Geometry check sheet. Reference: the model listing, model coordinates, mm. A direction names the side the tool comes from. Give positions to 0.01 mm unless a question says otherwise; leave off trailing zeros. Write each loop counter-clockwise with the first axis right and the second up, starting at its lowest first coordinate (ties: lowest second). Pieces come first, ordered by that corner, then holes. Notation, with made-up numbers: (38, -3) - (86, -3) arc R20 cw to (86, 34) - close; hole circle Ø9 at (73, -32.5). An arc over 180 degrees is marked (long way). One line per question, with ' | ' between items. Start each with the question number.
Q1. Section check B-B on y = 55.5. Record the boundary of the cut face in (x, z) (1 decimal).
Q2. Release check for a two-part mould opening along X. For faces 1 (the face through (127.808, 85.826, -0.876)), 2 (the face through (45.572, 109.968, 38.926)), 3 (the face through (66.636, 105.339, 41.819)) record: +X half, -X half, draft (parallel to the pull), parting line (faces both ways), or undercut.
Q3. Thickness scan on L1, parallel to Z at x = 125, y = 57; L2, parallel to X at y = 56, z = 0; L3, parallel to Y at x = 116.5, z = 8.5. Record the ranges inside material, lowest first. Write a range as [from, to].
Q4. Set-up check for faces 4 (the face through (121.238, 62.541, -2.724)), 5 (the face through (45.56, 101.81, 36.52)), 6 (the face through (119.16, 96.06, 1.78)): record each of +Z, -Z, +X, -X, +Y, -Y from which the full face is reachable in a straight line by a thin tool's end or side.
Q5. Section check A-A on x = 43. Record the boundary of the cut face in (y, z) (1 decimal).
Q6. Gauge pin test, flat ends, axial feed: P1, Ø1.5, axis at x = 92.5, y = 100, coming from the -Z side; P2, Ø10, axis at y = 105.25, z = 38.31, coming from the +X side; P3, Ø8, axis at x = 101, y = 102, coming from the -Z side. Record the tip position at first contact, or that the pin passes through.
```python
from build123d import *

# Parameters (mm, degrees)
PROFILE_R   = 4.7625
PROFILE_R_2 = 3.8735


with BuildPart() as part:
    # Tube: sweep along a curve in space
    with BuildLine() as tube_path:
        Line((28.2, 105.245573528, 38.306256052), (62.341451663, 105.245573528, 38.306256052))
        Line((62.341451663, 105.245573528, 38.306256052), (64.808223176, 105.218825972, 38.181995595))
        Line((64.808223176, 105.218825972, 38.181995595), (67.248866106, 105.138866619, 37.810530418))
        Line((67.248866106, 105.138866619, 37.810530418), (69.63752863, 105.006542417, 37.195795159))
        Line((69.63752863, 105.006542417, 37.195795159), (71.948909514, 104.823254972, 36.344301231))
        Line((71.948909514, 104.823254972, 36.344301231), (74.158526106, 104.590945705, 35.265067843))
        Line((74.158526106, 104.590945705, 35.265067843), (76.242973665, 104.312075287, 33.969526469))
        Line((76.242973665, 104.312075287, 33.969526469), (107.835723721, 99.58808025, 12.023380107))
        Line((107.835723721, 99.58808025, 12.023380107), (112.443681745, 98.197740878, 8.82242669))
        Line((112.443681745, 98.197740878, 8.82242669), (116.644976055, 95.506248168, 5.903965345))
        Line((116.644976055, 95.506248168, 5.903965345), (120.195899313, 91.669729365, 3.437289243))
        Line((120.195899313, 91.669729365, 3.437289243), (122.890470703, 86.910732024, 1.565484541))
        Line((122.890470703, 86.910732024, 1.565484541), (124.572384389, 81.505314539, 0.397130287))
        Line((124.572384389, 81.505314539, 0.397130287), (125.144076461, 75.767032634, 0))
        Line((125.144076461, 75.767032634, 0), (125.144076461, 49.4, 0))
    # Profile → Tube (sweep)
    with BuildSketch(Plane(origin=(28.2, 0, 0), x_dir=(0, 0, -1), z_dir=(1, 0, 0))):
        with Locations((-38.306256052, 105.245573528)):
            Circle(PROFILE_R)
        with Locations((-38.306256052, 105.245573528)):
            Circle(PROFILE_R_2, mode=Mode.SUBTRACT)
    sweep(path=tube_path.line, transition=Transition.RIGHT)


solid = part.part
```
Working result:
1) outline: circle Ø9.5 at (125.1, 0); hole circle Ø7.7 at (125.1, 0)
2) face 1: parting line | face 2: draft | face 3: undercut
3) L1: z = [-4.76, -3.87], [3.87, 4.76] | L2: x = [120.38, 121.27], [129.02, 129.91] | L3: y = [91.18, 92.53], [100.06, 101.21]
4) face 4: -Y | face 5: -X | face 6: none
5) outline: circle Ø9.5 at (105.2, 38.3); hole circle Ø7.7 at (105.2, 38.3)
6) P1: stops at z = 16.55 | P2: stops at x = 85.25 | P3: stops at z = 8.48
